```python
from build123d import *

# Parameters (mm, degrees)
F0_W      = 117.475
F0_H      = 25.4
F1_DEPTH  = 15.875
F3_D      = 6.35
F3_DEPTH  = 177.8
F3_TIP    = 1.9077324654
F5_D      = 10.16
F5_DEPTH  = 177.8
F5_TIP    = 3.0523719447
F7_D      = 7.62
F7_DEPTH  = 177.8
F7_TIP    = 2.2892789585
F9_D      = 6.35
F9_DEPTH  = 177.8
F9_TIP    = 1.9077324654
F11_D     = 3.556
F11_DEPTH = 25.4
F11_TIP   = 1.0683301806


# Not quite as in the source:
# - a feature names something its author has since deleted; it is built from what else it names


with BuildPart() as f1:
    # F0 (on Front) → F1 (new body)
    with BuildSketch(Plane.XZ):
        with Locations((58.7375, 12.7)):
            Rectangle(F0_W, F0_H)
    extrude(amount=F1_DEPTH)

    # F3
    with Locations(Plane(origin=(0, 0, 0), x_dir=(1, 0, 0), z_dir=(0, 0, -1))):
        with Locations((45.984800905, 6.7214882001)):
            Hole(F3_D / 2, depth=F3_DEPTH)
            with Locations((0, 0, -(F3_DEPTH + F3_TIP / 2))):  # 118° drill point
                Cone(0, F3_D / 2, F3_TIP, mode=Mode.SUBTRACT)

    # F5
    with Locations(Plane(origin=(0, 0, 0), x_dir=(1, 0, 0), z_dir=(0, 0, -1))):
        with Locations((59.3467913568, 7.1263969876)):
            Hole(F5_D / 2, depth=F5_DEPTH)
            with Locations((0, 0, -(F5_DEPTH + F5_TIP / 2))):  # 118° drill point
                Cone(0, F5_D / 2, F5_TIP, mode=Mode.SUBTRACT)

    # F7
    with Locations(Plane(origin=(0, 0, 0), x_dir=(1, 0, 0), z_dir=(0, 0, -1))):
        with Locations((109.7984462976, 7.531305775)):
            Hole(F7_D / 2, depth=F7_DEPTH)
            with Locations((0, 0, -(F7_DEPTH + F7_TIP / 2))):  # 118° drill point
                Cone(0, F7_D / 2, F7_TIP, mode=Mode.SUBTRACT)

    # F9
    with Locations(Plane(origin=(0, 0, 0), x_dir=(1, 0, 0), z_dir=(0, 1, 0))):
        with Locations((72.8548616171, -10.5120344087)):
            Hole(F9_D / 2, depth=F9_DEPTH)
            with Locations((0, 0, -(F9_DEPTH + F9_TIP / 2))):  # 118° drill point
                Cone(0, F9_D / 2, F9_TIP, mode=Mode.SUBTRACT)

    # F11
    with Locations(Plane(origin=(0, 0, 0), x_dir=(1, 0, 0), z_dir=(0, 1, 0))):
        with Locations((102.7114540339, -2.0629046485)):
            Hole(F11_D / 2, depth=F11_DEPTH)
            with Locations((0, 0, -(F11_DEPTH + F11_TIP / 2))):  # 118° drill point
                Cone(0, F11_D / 2, F11_TIP, mode=Mode.SUBTRACT)


solid = f1.part
```
Work out the finished part from the listing and answer in its coordinate system (mm). Coordinates: 2 decimals unless noted, no trailing zeros. Loops run counter-clockwise (first coordinate to the right, second up) from the corner with the lowest first, then second, coordinate; pieces in that order, holes last. Notation, with made-up numbers: (49, 70) -> (73, 70) arc R34 ccw to (73, 103) -> close; hole circle Ø11 at (-9.75, 33). An arc over 180 degrees is marked (long way). Answer as CSV lines item,"result".
Q1. The part is cut by section B-B on z = 23.5. Write down the section's boundary in (x, y) (3 decimals).
Findings:
outline,"(0, -15.875) -> (117.475, -15.875) -> (117.475, 0) -> (0, 0) -> close; hole circle Ø6.35 at (45.985, -6.721); hole circle Ø10.16 at (59.347, -7.126); hole circle Ø7.62 at (109.798, -7.531)"
Q2. Find the intervals of material crossed by probe 1 along X at (y, z) = (-5.25, 7.25) (3 decimals); probe 2 along X at (y, z) = (-5, 16) (3 decimals); probe 3 along Y at (x, z) = (108.5, 6.5) (3 decimals), in increasing order.
Findings:
probe 1,"x = 0 to 43.171, 48.798 to 54.626, 64.068 to 106.747, 112.85 to 117.475"
probe 2,"x = 0 to 43.317, 48.653 to 54.733, 63.96 to 106.951, 112.646 to 117.475"
probe 3,"y = -15.875 to -11.113, -3.949 to 0"
Q3. The part is cut by section C-C on x = 109. Write down the section's boundary in (y, z) (3 decimals), and give its area (3 significant figures).
Findings:
outline,"(-15.875, 0) -> (-11.257, 0) -> (-11.257, 25.4) -> (-15.875, 25.4) -> close; (-3.806, 0) -> (0, 0) -> (0, 25.4) -> (-3.806, 25.4) -> close"
area,"214 mm²"
Q4. For a pull along X with two mould halves and no side action, classify faces 1 (the face through (0, -8, 13)), 2 (the face through (49.157, -6.861, 12.878)), 3 (the face through (58, 0, 13)) as +X half, -X half, draft (parallel to the pull), parting line (faces both ways), or undercut.
Findings:
face 1,"-X half"
face 2,"undercut"
face 3,"draft"
Q5. The part is cut by section A-A on x = 73.5. Write down the section's boundary in (y, z) (3 decimals), and give its area (3 significant figures).
Findings:
outline,"(-15.875, 0) -> (0, 0) -> (0, 7.403) -> (-15.875, 7.403) -> close; (-15.875, 13.621) -> (0, 13.621) -> (0, 25.4) -> (-15.875, 25.4) -> close"
area,"305 mm²"
